```python
from build123d import *

# Parameters (mm, degrees)
PAD005_DEPTH    = 30
POCKET007_DEPTH = 10
SKETCH019_W     = 20
SKETCH019_H     = 2
PAD006_DEPTH    = 10
PAD018_DEPTH    = 10
SKETCH016_R     = 2
POCKET005_DEPTH = 2.001
SKETCH017_R     = 4
POCKET006_DEPTH = 48.001
FILLET002_R     = 8
FILLET003_R     = 0.4


with BuildPart() as rearhullleftbody:
    # Sketch015 → Pad005 (new body)
    with BuildSketch(Plane.YZ):
        Polygon((0, 40), (0, 0), (75, 0), align=None)
    extrude(amount=PAD005_DEPTH)

    # Sketch018 (on Face5 of Pad005) → Pocket007 (cut)
    with BuildSketch(Plane.YZ.offset(30)):
        Polygon((0, 20), (0, 0), (50, 0), (50, 5), align=None)
    extrude(amount=-POCKET007_DEPTH, mode=Mode.SUBTRACT)

    # Sketch019 (on Face6 of Pocket007) → Pad006 (join)
    with BuildSketch(Plane.YZ.offset(30)):
        with Locations((10, 26)):
            Rectangle(SKETCH019_W, SKETCH019_H)
    extrude(amount=PAD006_DEPTH)

    # Pad006 Face2 → Pad018 (add)
    with BuildSketch(Plane(origin=(12.142857, 41.071429, 0), x_dir=(0, -1, 0), z_dir=(0, 0, -1))):
        Polygon((41.071429, 12.142857), (-33.928571, 12.142857), (-33.928571, -17.857143), (-8.928571, -17.857143), (-8.928571, -7.857143), (41.071429, -7.857143), align=None)
    extrude(amount=PAD018_DEPTH)

    # Sketch016 (on DatumPlane) → Pocket005 (cut, through all)
    with BuildSketch(Plane(origin=(0, 0, -8), x_dir=(-1, 0, 0), z_dir=(0, 0, -1))):
        with Locations((-8, 38.5)):
            Circle(SKETCH016_R)
        with Locations((-8, 8.5)):
            Circle(SKETCH016_R)
    extrude(amount=POCKET005_DEPTH, mode=Mode.SUBTRACT)

    # Sketch017 (on DatumPlane) → Pocket006 (cut, through all)
    with BuildSketch(Plane(origin=(0, 0, -8), x_dir=(-1, 0, 0), z_dir=(0, 0, -1))):
        with Locations((-8, 8.5)):
            Circle(SKETCH017_R)
        with Locations((-8, 38.5)):
            Circle(SKETCH017_R)
    extrude(amount=-POCKET006_DEPTH, mode=Mode.SUBTRACT)

    # Fillet002
    fillet002_edges = [rearhullleftbody.edges().sort_by_distance(p)[0] for p in [
        (0, 75, -5),
    ]]
    fillet(fillet002_edges, radius=FILLET002_R)

    # Fillet003
    fillet003_edges = [rearhullleftbody.edges().sort_by_distance(p)[0] for p in [
        (30, 75, -5),
        (0, 33.5, -10),
        (0, 0, 15),
        (10, 0, -10),
        (15, 0, 40),
        (19, 75, -10),
        (19, 75, 0),
        (0, 33.5, 22.133333),
        (30, 62.5, -10),
    ]]
    fillet(fillet003_edges, radius=FILLET003_R)


with BuildPart() as rearhullleftbody_1:
    # Body006 placement: moved
    add(rearhullleftbody.part.moved(Location((-77.5, 25, 13))))


with BuildPart() as part_mirroring001:
    # Part__Mirroring001: instance of RearHullLeftBody
    add(rearhullleftbody_1.part.mirror(Plane(origin=(0, 0, 0), x_dir=(0, -1, 0), z_dir=(1, 0, 0))))


solid = part_mirroring001.part
```
Here's how the part is built. I have some questions about the finished solid (model axes, mm). A direction names the side the tool comes from. Coordinates: 2 decimals unless noted, no trailing zeros. Write each loop counter-clockwise with the first axis right and the second up, starting at its lowest first coordinate (ties: lowest second). Pieces come first, ordered by that corner, then holes. Notation, with made-up numbers: (33, 46.5) -> (89, 46.5) arc R26 ccw to (89, 80.5) -> close; hole circle Ø9 at (-3, -4). An arc over 180 degrees is marked (long way). Use a Markdown table: item, result. Add a question column.
(1) We'd pull the mould along Y, two halves only. Please class faces 4 (the flat face through (57.5, 50, 15)), 5 (the cylindrical face through (70.423, 31.726, 4.014)), 6 (the flat face through (61, 25, 34)): +Y half, -Y half, draft (parallel to the pull), parting line (faces both ways), or undercut.
(2) If we section it at A-A, the plane z = 7: Write out the boundary of the cut face in (x, y).
(3) I'm going to push flat-ended pins straight in: P1, Ø4, axis at x = 68, y = 63, coming from the +Z side; P2, Ø5, axis at x = 51.5, y = 56, coming from the +Z side; P3, Ø5, axis at x = 43, y = 40, coming from the +Z side; P4, Ø7, axis at x = 69.5, y = 33.5, coming from the -Z side. Where does each tip first touch, or does it pass through?
(4) If we section it at D-D, the plane z = 15.5: State how many separate pieces and enclosed holes the cut face has, and give its area (3 significant figures).
(5) For faces 1 (the flat face through (43, 45, 39)), 2 (the flat face through (43, 35, 40)), 3 (the cylindrical face through (71.346, 59.951, 19.618)), which set-ups out of +Z, -Z, +X, -X, +Y, -Y let a thin tool reach every point of the face, with its end or its side?
(6) If we section it at C-C, the plane x = 51.5: Write out the boundary of the cut face in (y, z).
(7) Please list where these lines run through material, in increasing order: line 1 (X direction, y = 63.5, z = 26.5); line 2 (X direction, y = 63.5, z = 16.25); line 3 (Y direction, x = 69, z = 4).
(8) If we section it at B-B, the plane x = 60.5: Write out the boundary of the cut face in (y, z).
Outcome:
| question | item | result |
|---|---|---|
| 1 | face 4 | draft |
| 1 | face 5 | undercut |
| 1 | face 6 | -Y half |
| 2 | outline | (47.5, 75) -> (57.5, 75) -> (57.5, 25) -> (77.1, 25) arc R0.4 ccw to (77.5, 25.4) -> (77.5, 92) arc R8 ccw to (69.5, 100) -> (47.9, 100) arc R0.4 ccw to (47.5, 99.6) -> close; hole circle Ø8 at (69.5, 33.5); hole circle Ø8 at (69.5, 63.5) |
| 3 | P1 | stops at z = 5 |
| 3 | P2 | stops at z = 37.8 |
| 3 | P3 | stops at z = 40 |
| 3 | P4 | stops at z = 3 |
| 4 | separate pieces | 1 |
| 4 | enclosed holes | 2 |
| 4 | area | 1,510 mm^2 |
| 5 | face 1 | +Z, -Z, -X, +Y |
| 5 | face 2 | +Z, -X, +Y, -Y |
| 5 | face 3 | +Z |
| 6 | outline | (25, 33) -> (75, 18) -> (75, 3) -> (99.6, 3) arc R0.4 ccw to (100, 3.4) -> (100, 12.76) arc R0.4 ccw to (99.79, 13.11) -> (25.59, 52.69) arc R0.4 ccw to (25, 52.33) -> close |
| 7 | line 1 | x = 47.5 to 65.5, 73.5 to 77.5 |
| 7 | line 2 | x = 57.5 to 65.5, 73.5 to 77.5 |
| 7 | line 3 | y = 25 to 31.56, 35.44 to 61.56, 65.44 to 100 |
| 8 | outline | (25, 3.4) arc R0.4 ccw to (25.4, 3) -> (99.6, 3) arc R0.4 ccw to (100, 3.4) -> (100, 12.76) arc R0.4 ccw to (99.79, 13.11) -> (25.59, 52.69) arc R0.4 ccw to (25, 52.33) -> close |
